The model under review builds one solid part; all positions refer to its coordinate system, in mm. A direction names the side the tool comes from. Give positions to 0.01 mm unless a question says otherwise; leave off trailing zeros. Order: outer loops, then holes, each group sorted by start corner. A loop starts at its lowest first (then second) coordinate and runs counter-clockwise, first axis right, second up. Notation, with made-up numbers: (12.5, 43) - (60.5, 43) arc R21 cw to (60.5, 57) - close; hole circle Ø4 at (59.25, 28.25). An arc over 180 degrees is marked (long way). Write item = value, one per line. Start each with the question number.
1. For P1, Ø3, axis at y = 41, z = 23, coming from the -X side; P2, Ø7.5, axis at x = 24, z = 31.5, coming from the +Y side; P3, Ø6, axis at y = 14.5, z = 33, coming from the -X side, all flat-tipped, find the tip position at first contact; note any pin that passes through.
2. Machinability: for faces 4 (the flat face through (35, 35, 25)), 5 (the flat face through (25, 10, 30)), 6 (the flat face through (60, 47, 30)), which of the approach directions +Z, -Z, +X, -X, +Y, -Y give a long, thin tool a straight path to every point of the face, cutting with its end or side? Answer none if there is none.
3. We need section C-C, the plane z = 27.5. Give the boundary of the cut face in (x, y).
4. We need section A-A, the plane x = 40. Give the boundary of the cut face in (y, z), and give its area (3 significant figures).
5. Mouldability with a two-part tool opening along X and no side actions: class faces 1 (the flat face through (23, 59, 20)), 2 (the flat face through (47.325, 59.86, 24.93)), 3 (the cylindrical face through (61.63, 42.32, 25.07)) as pulls with the +X half, pulls with the -X half, needs draft (parallel to the pull), parting line crosses it, or undercut.
6. Wall thickness on probe 1 along X at (y, z) = (35, 23); probe 2 along Z at (x, y) = (55, 65); probe 3 along Z at (x, y) = (25, 14): over which ranges is each line inside the solid? List them lowest first.
7. We need section B-B, the plane y = 43.5. Give the boundary of the cut face in (x, z).
8. We need section D-D, the plane z = 16. Give the boundary of the cut face in (x, y).
Autodesk Fusion 360 part; units mm, degrees
sketch "Sketch1" plane through (0, 0, 0) normal (0, 0, 1) x (1, 0, 0) in component "block"
  line L0 (0, 0) -> (75, 0)
  line L1 (75, 0) -> (75, 75)
  line L2 (75, 75) -> (75, 90)
  line L3 (0, 0) -> (0, 70)
  line L4 (0, 70) -> (25, 90)
  line L5 (25, 90) -> (75, 90)
extrude "Extrude1" add sketch "Sketch1" along normal blind 20 in component "block"
sketch "Sketch2" plane through (0, 0, 20) normal (0, 0, 1) x (-1, 0, 0) in component "block"
  line L0 (0, 0) -> (-75, 0)
  line L1 (-75, 0) -> (-75, -90)
  line L2 (-75, -90) -> (-25, -90)
  line L3 (-25, -90) -> (0, -70)
  line L4 (0, -70) -> (0, 0)
  line L5 (-75, -20) -> (-35, -20)
  line L6 (-35, -20) -> (-35, -50)
  line L7 (-35, -50) -> (-60, -70)
  line L8 (-60, -70) -> (-60, -90)
extrude "Extrude2" add sketch "Sketch2" along normal blind 10 contours L1 L2 L5 L6 L7 L8 in component "block"
sketch "Sketch3" plane through (0, 0, 20) normal (0, 0, 1) x (-1, 0, 0) in component "block"
  line L0 (-60, -70) -> (-60, -90)
  line L1 (-60, -90) -> (-25, -90)
  line L2 (-25, -90) -> (0, -70)
  line L3 (0, -70) -> (0, 0)
  line L4 (0, 0) -> (-75, 0)
  line L5 (-75, 0) -> (-75, -20)
  line L6 (-75, -20) -> (-35, -20)
  line L7 (-35, -20) -> (-35, -50)
  line L8 (-35, -50) -> (-60, -70)
  line L9 (-35, -20) -> (-10, -20)
  line L10 (-10, -20) -> (0, -10)
extrude "Extrude3" add sketch "Sketch3" along normal blind 20 contours L3 L4 L5 L6 L9 L10 in component "block"
sketch "Sketch4" plane through (0, 0, 30) normal (0, 0, 1) x (-1, 0, 0) in component "block"
  line L0 (-75, -20) -> (-75, -90)
  line L1 (-75, -90) -> (-60, -90)
  line L2 (-60, -90) -> (-60, -70)
  line L3 (-60, -70) -> (-35, -50)
  line L4 (-35, -50) -> (-35, -20)
  line L5 (-35, -20) -> (-75, -20)
  circle A0 centre (-60, -35) radius 7.5
  dimension "d7" = 15
extrude "Extrude4" cut sketch "Sketch4" against normal blind 10 contours A0 in component "block"
sketch "Sketch5" plane through (0, 20, 0) normal (0, 1, 0) x (-1, 0, 0) in component "block"
  line L0 (-75, 30) -> (-35, 30)
  line L1 (-35, 30) -> (-35, 20)
  line L2 (-35, 20) -> (-10, 20)
  line L3 (-10, 20) -> (-10, 40)
  line L4 (-10, 40) -> (-75, 40)
  line L5 (-75, 40) -> (-75, 30)
  circle A0 centre (-25, 30) radius 7.5
  dimension "d11" = 15
extrude "Extrude5" cut sketch "Sketch5" against normal blind 10 contours A0 in component "block"
component "block" placed x (1, 0, 0) y (0, 1, 0) z (0, 0, 1) at (0, 0, 0)
Model answer:
q1.P1 = 35
q1.P2 = 10
q1.P3 = 1.5
q2.face_4 = +Z, -X, +Y
q2.face_5 = +Y
q2.face_6 = +Z, +X, -X, +Y
q3.outline = (0, 0) - (75, 0) - (75, 90) - (60, 90) - (60, 70) - (35, 50) - (35, 20) - (32.07, 20) - (32.07, 10) - (17.93, 10) - (17.93, 20) - (10, 20) - (0, 10) - close; hole circle Ø15 at (60, 35)
q4.outline = (0, 0) - (90, 0) - (90, 20) - (54, 20) - (54, 30) - (20, 30) - (20, 40) - (0, 40) - close
q4.area = 2,540 mm2
q5.face_1 = needs draft
q5.face_2 = pulls with the -X half
q5.face_3 = undercut
q6.probe_1 = 35 to 52.5, 67.5 to 75
q6.probe_2 = 0 to 30
q6.probe_3 = 0 to 22.5, 37.5 to 40
q7.outline = (0, 0) - (75, 0) - (75, 30) - (35, 30) - (35, 20) - (0, 20) - close
q8.outline = (0, 0) - (75, 0) - (75, 90) - (25, 90) - (0, 70) - close
